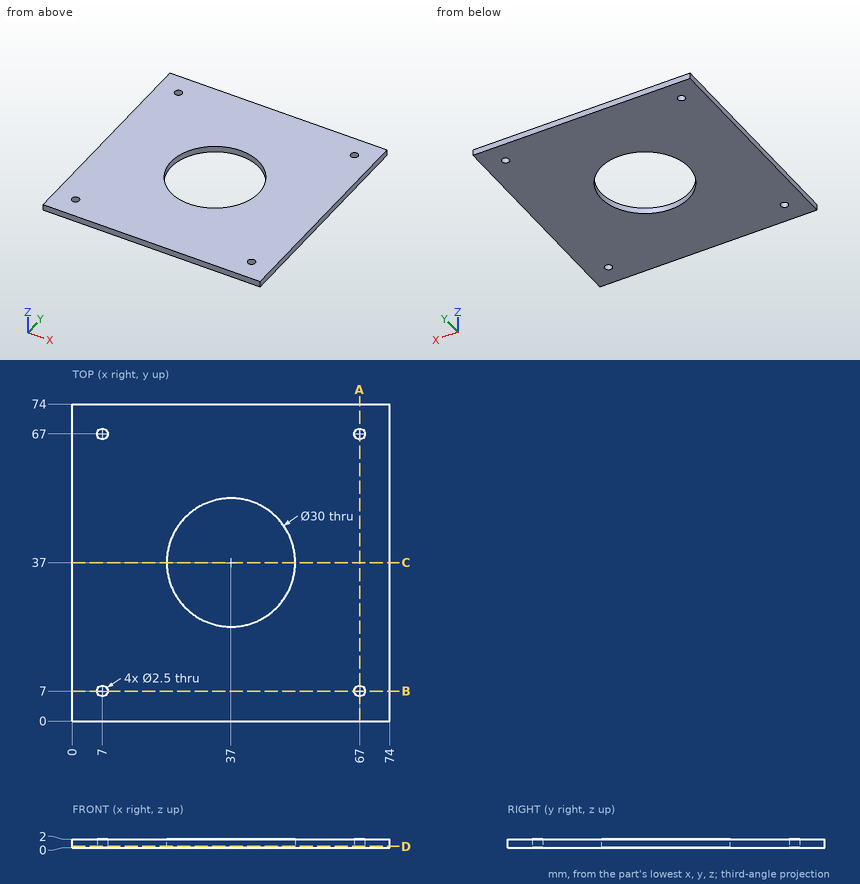
Check sheet for the drawn part. Datum: minimum x, y, z corner. Units: mm. Round coordinates to 2 decimals unless told otherwise and drop trailing zeros. Write each loop counter-clockwise with the first axis right and the second up, starting at its lowest first coordinate (ties: lowest second). Pieces come first, ordered by that corner, then holes. Notation, with made-up numbers: (89, -16.75) -> (114, -16.75) arc R14 cw to (114, -4.75) -> close; hole circle Ø1 at (65.25, 78). An arc over 180 degrees is marked (long way). One line per item, written item: value. Start each with the question number.
(1) Cross-section at C-C, the plane y = 37. Record the cut outline in (x, z), and give its area (3 significant figures).
(2) Cross-section at A-A, the plane x = 67. Record the cut outline in (y, z), and give its area (3 significant figures).
(3) Scan lines: line 1 (Y direction, x = 67, z = 0.95); line 2 (X direction, y = 7.5, z = 0.1). Record each from-to range of solid material in increasing order. Write a range as [from, to].
(4) Cross-section at D-D, the plane z = 0.3. Record the cut outline in (x, y), and give its area (3 significant figures).
Answer:
1. outline: (0, 0) -> (22, 0) -> (22, 2) -> (0, 2) -> close; (52, 0) -> (74, 0) -> (74, 2) -> (52, 2) -> close
1. area: 88.0 mm²
2. outline: (0, 0) -> (5.75, 0) -> (5.75, 2) -> (0, 2) -> close; (8.25, 0) -> (65.75, 0) -> (65.75, 2) -> (8.25, 2) -> close; (68.25, 0) -> (74, 0) -> (74, 2) -> (68.25, 2) -> close
2. area: 138 mm²
3. line 1: [0, 5.75], [8.25, 65.75], [68.25, 74]
3. line 2: [0, 5.85], [8.15, 65.85], [68.15, 74]
4. outline: (0, 0) -> (74, 0) -> (74, 74) -> (0, 74) -> close; hole circle Ø2.5 at (7, 7); hole circle Ø2.5 at (7, 67); hole circle Ø30 at (37, 37); hole circle Ø2.5 at (67, 7); hole circle Ø2.5 at (67, 67)
4. area: 4,750 mm²
